from build123d import *

# Parameters (mm, degrees)
SKETCH1_W                       = 19.05
SKETCH1_H                       = 6.35
BOSS_EXTRUDE1_DEPTH             = 25.4
SKETCH2_R                       = 3.175
BOSS_EXTRUDE3_DEPTH             = 25.4
CUT_EXTRUDE5_DEPTH              = 11.43
CUT_EXTRUDE6_DEPTH              = 26.4
CUT_EXTRUDE9_DEPTH              = 11.43
F_9_64_0_14063_DIAMETER_HOLE3_D = 3.572002


with BuildPart() as part:
    # Sketch1 → Boss-Extrude1 (new body)
    with BuildSketch(Plane.XY):
        Polygon((24.387960916, 24.466176471), (24.387960916, 21.291176471), (5.337960916, 21.291176471), align=None)
        with Locations((14.862960916, 18.116176471)):
            Rectangle(SKETCH1_W, SKETCH1_H)
    extrude(amount=-BOSS_EXTRUDE1_DEPTH)

    # Sketch2 → Boss-Extrude3 (add)
    with BuildSketch(Plane.XY):
        with Locations((24.387960916, 21.291176471)):
            Circle(SKETCH2_R)
    extrude(amount=-BOSS_EXTRUDE3_DEPTH)

    # Sketch9 → Cut-Extrude5 (cut)
    with BuildSketch(Plane.XY):
        with BuildLine():
            Line((23.358231186, 24.294554849), (7.877960916, 21.714509804))
            Line((7.877960916, 21.714509804), (7.877960916, 17.481176471))
            Line((7.877960916, 17.481176471), (19.942960916, 17.481176471))
            Line((19.942960916, 17.481176471), (21.212960916, 18.751176471))
            Line((21.212960916, 18.751176471), (21.212960916, 21.291176471))
            ThreePointArc((21.212960916, 21.291176471), (21.804357145, 23.136607736), (23.358231186, 24.294554849))
        make_face()
    extrude(amount=-CUT_EXTRUDE5_DEPTH, mode=Mode.SUBTRACT)

    # Sketch10 → Cut-Extrude6 (cut, through all)
    with BuildSketch(Plane.XY):
        Polygon((24.387960916, 18.116176471), (21.212960916, 14.941176471), (24.387960916, 14.941176471), align=None)
    extrude(amount=-CUT_EXTRUDE6_DEPTH, mode=Mode.SUBTRACT)

    # Sketch17 → Cut-Extrude9 (cut)
    with BuildSketch(Plane(origin=(0, 0, -25.4), x_dir=(-1, 0, 0), z_dir=(0, 0, -1))):
        with BuildLine():
            Line((-7.877960916, 21.714509804), (-23.358231186, 24.294554849))
            ThreePointArc((-23.358231186, 24.294554849), (-21.804357145, 23.136607736), (-21.212960916, 21.291176471))
            Line((-21.212960916, 21.291176471), (-21.212960916, 18.751176471))
            Line((-21.212960916, 18.751176471), (-19.942960916, 17.481176471))
            Line((-19.942960916, 17.481176471), (-7.877960916, 17.481176471))
            Line((-7.877960916, 17.481176471), (-7.877960916, 21.714509804))
        make_face()
    extrude(amount=-CUT_EXTRUDE9_DEPTH, mode=Mode.SUBTRACT)

    # 9/64 (0.14063) Diameter Hole3 (through all)
    with Locations(Plane(origin=(24.387960916, 21.291176471, 0), x_dir=(1, 0, 0), z_dir=(0, 0, 1))):
        with Locations((0, 0)):
            Hole(F_9_64_0_14063_DIAMETER_HOLE3_D / 2)


solid = part.part
Verification items for the finished model (mm, model axes). A direction names the side the tool comes from. Round coordinates to 2 decimals unless told otherwise and drop trailing zeros. Loops run counter-clockwise (first coordinate to the right, second up) from the corner with the lowest first, then second, coordinate; pieces in that order, holes last. Notation, with made-up numbers: M 28.5,87.25 L 38.5,87.25 A21 ccw 38.5,117.25 Z; hole C 33.25,-7 d7. An arc over 180 degrees is marked long. Write each question's results on one line, items separated by ' | '.
1) Section check B-B on y = 22.5. Record the boundary of the cut face in (x, z).
Checks:
outline: M 12.59,-13.97 L 21.45,-13.97 L 21.45,-25.4 L 23.07,-25.4 L 23.07,0 L 21.45,0 L 21.45,-11.43 L 12.59,-11.43 Z; M 25.7,-25.4 L 27.32,-25.4 L 27.32,0 L 25.7,0 Z
2) Mould release check, pull along X, two halves, no side actions. Record for faces 1 (the flat face through (22.82, 16.55, -12.52)), 2 (the flat face through (16, 17, -25.4)), 3 (the flat face through (7.878, 20, -6)), 4 (the flat face through (10.3, 22.12, -12.64)): released by +X, released by -X, zero draft, split by the parting line, or undercut.
Checks:
face 1: released by +X | face 2: zero draft | face 3: undercut | face 4: released by -X
3) Section check C-C on x = 8.5. Record the boundary of the cut face in (y, z).
Checks:
outline: M 14.94,-25.4 L 17.48,-25.4 L 17.48,-13.97 L 21.82,-13.97 L 21.82,-11.43 L 17.48,-11.43 L 17.48,0 L 14.94,0 Z
4) Gauge pin test, flat ends, axial feed: P1, Ø3.5, axis at x = 17, y = 20, coming from the +Z side; P2, Ø1.3, axis at y = 20, z = -21.5, coming from the +X side; P3, Ø1.5, axis at y = 21, z = -12, coming from the +X side; P4, Ø10, axis at x = 7.5, z = -22.5, coming from the +Y side. Record the tip position at first contact, or that the pin passes through.
Checks:
P1: stops at z = -11.43 | P2: stops at x = 27.5 | P3: stops at x = 27.56 | P4: stops at y = 21.71
5) Scan lines: L1, parallel to X at y = 20, z = -9.75; L2, parallel to Y at x = 19, z = -9.5; L3, parallel to Z at x = 10.75, y = 17.75. Record each from-to range of solid material in increasing order. Write a range as from..to.
Checks:
L1: x = 5.34..7.88, 21.21..23.15, 25.62..27.29 | L2: y = 14.94..17.48 | L3: z = -13.97..-11.43
6) Section check D-D on z = -12. Record the boundary of the cut face in (x, y) (3 decimals), then the cut area to 3 significant figures.
Checks:
outline: M 5.338,14.941 L 21.213,14.941 L 24.388,18.116 A3.175 ccw long 23.358,24.295 L 5.338,21.291 Z; hole C 24.388,21.291 d3.572 | area: 152 mm2
7) Access from +Z, -Z, +X, -X, +Y, -Y to the whole of each face (thin tool, end or side, straight path). Record for faces 5 (the flat face through (20.57, 18.11, -5.63)), 6 (the flat face through (20.59, 18.13, -19.77)), 7 (the flat face through (16, 17, 0)).
Checks:
face 5: +Z, +Y | face 6: -Z, +Y | face 7: +Z, +X, -X, +Y, -Y
